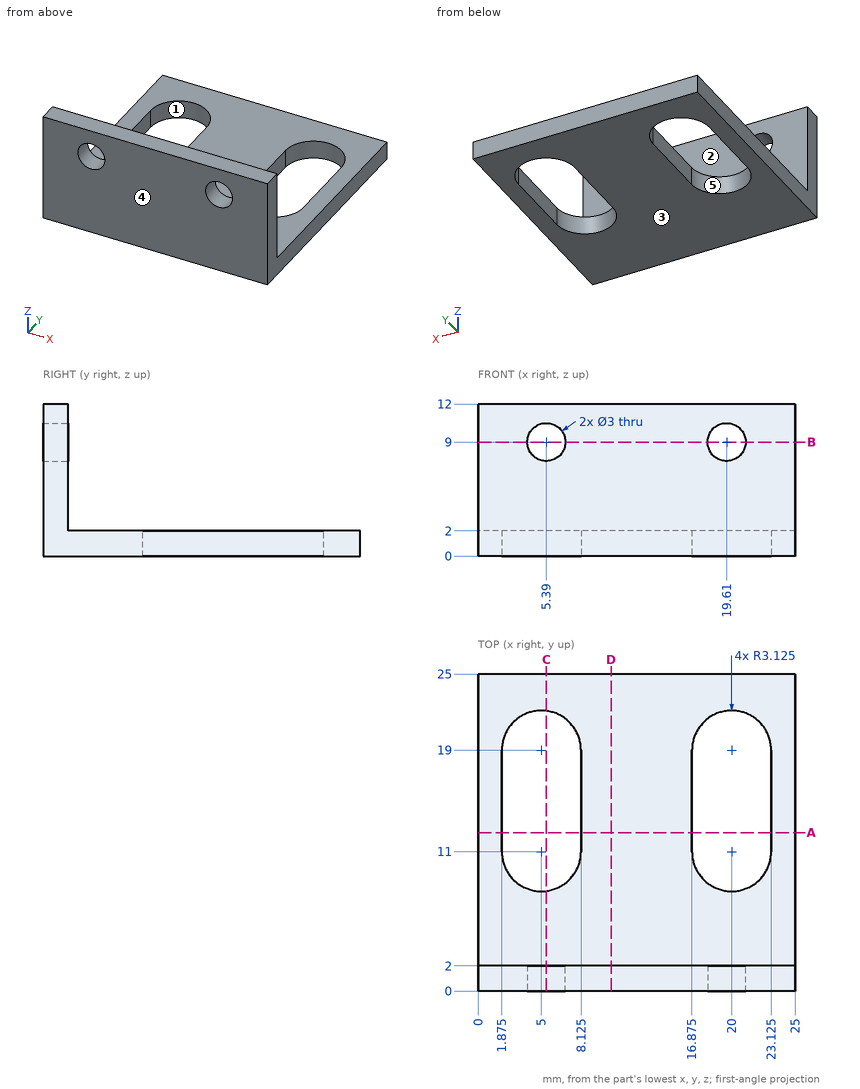
The figure shows three views and two pictorial views of one solid part (mm, origin at its lowest corner). Answer the questions. A direction names the side the tool comes from. Give positions to 0.01 mm unless a question says otherwise; leave off trailing zeros. Order: outer loops, then holes, each group sorted by start corner. A loop starts at its lowest first (then second) coordinate and runs counter-clockwise, first axis right, second up. Notation, with made-up numbers: (74.25, 12) -> (93.25, 12) arc R23 cw to (93.25, 48) -> close; hole circle Ø9 at (74, 29.25). An arc over 180 degrees is marked (long way). Answer as a JSON object with one key per item and string values. Group by question number.
Item 1: A tool of negligible diameter and unlimited length cuts with its end or side. For the marked faces 1, 2 and 3, from which of +Z, -Z, +X, -X, +Y, -Y can it reach the whole face along a straight path? Write none if from no direction.
Item 2: The part is cut by section B-B on z = 9. Write down the section's boundary in (x, y).
Item 3: Flat-ended cylindrical pins translate along their axes: pin 1 (11.5 mm diameter, centred on x = 14.5, y = 9.5, fed in from +Z); pin 2 (2.5 mm diameter, centred on x = 19.61, z = 9, fed in from +Y). Find the tip coordinate at first contact, or state that the pin passes through.
Item 4: Consider L1, parallel to X at y = 1.5, z = 9.25; L2, parallel to Z at x = 19.61, y = 0.95; L3, parallel to Y at x = 1, z = 4.75. Determine where each line is inside the solid, lowest interval first. Write a range as from..to.
Item 5: The part is cut by section C-C on x = 5.39. Write down the section's boundary in (y, z).
Item 6: The part is cut by section D-D on x = 10.5. Write down the section's boundary in (y, z), and give its area (3 significant figures).
Item 7: Determine the mould class of the marked faces 4 and 5 for opening direction X: pulls with the +X half, pulls with the -X half, needs draft (parallel to the pull), parting line crosses it, or undercut.
Item 8: The part is cut by section A-A on y = 12.5. Write down the section's boundary in (x, z) (3 decimals), and give its area (3 significant figures).
Result set:
{
 "1": {"face 1": "+Z, -Z", "face 2": "+Z, +X, -X, +Y", "face 3": "-Z, +X, -X, +Y, -Y"},
 "2": {"outline": "(0, 0) -> (3.89, 0) -> (3.89, 2) -> (0, 2) -> close; (6.89, 0) -> (18.11, 0) -> (18.11, 2) -> (6.89, 2) -> close; (21.11, 0) -> (25, 0) -> (25, 2) -> (21.11, 2) -> close"},
 "3": {"pin 1": "z = 2", "pin 2": "through"},
 "4": {"L1": "0..3.91, 6.87..18.13, 21.09..25", "L2": "0..7.5, 10.5..12", "L3": "0..2"},
 "5": {"outline": "(0, 0) -> (7.9, 0) -> (7.9, 2) -> (2, 2) -> (2, 7.5) -> (0, 7.5) -> close; (0, 10.5) -> (2, 10.5) -> (2, 12) -> (0, 12) -> close; (22.1, 0) -> (25, 0) -> (25, 2) -> (22.1, 2) -> close"},
 "6": {"outline": "(0, 0) -> (25, 0) -> (25, 2) -> (2, 2) -> (2, 12) -> (0, 12) -> close", "area": "70.0 mm²"},
 "7": {"face 4": "needs draft", "face 5": "undercut"},
 "8": {"outline": "(0, 0) -> (1.875, 0) -> (1.875, 2) -> (0, 2) -> close; (8.125, 0) -> (16.875, 0) -> (16.875, 2) -> (8.125, 2) -> close; (23.125, 0) -> (25, 0) -> (25, 2) -> (23.125, 2) -> close", "area": "25.0 mm²"}
}
